Check sheet for the drawn part. Datum: minimum x, y, z corner. Units: mm. A direction names the side the tool comes from. Give positions to 0.01 mm unless a question says otherwise; leave off trailing zeros. Order: outer loops, then holes, each group sorted by start corner. A loop starts at its lowest first (then second) coordinate and runs counter-clockwise, first axis right, second up. Notation, with made-up numbers: M 26.25,0.5 L 31.25,0.5 A14 cw 31.25,4.5 Z; hole C 47,6 d10. An arc over 180 degrees is marked long. Answer in a Markdown table with one row per item. Add a question column.
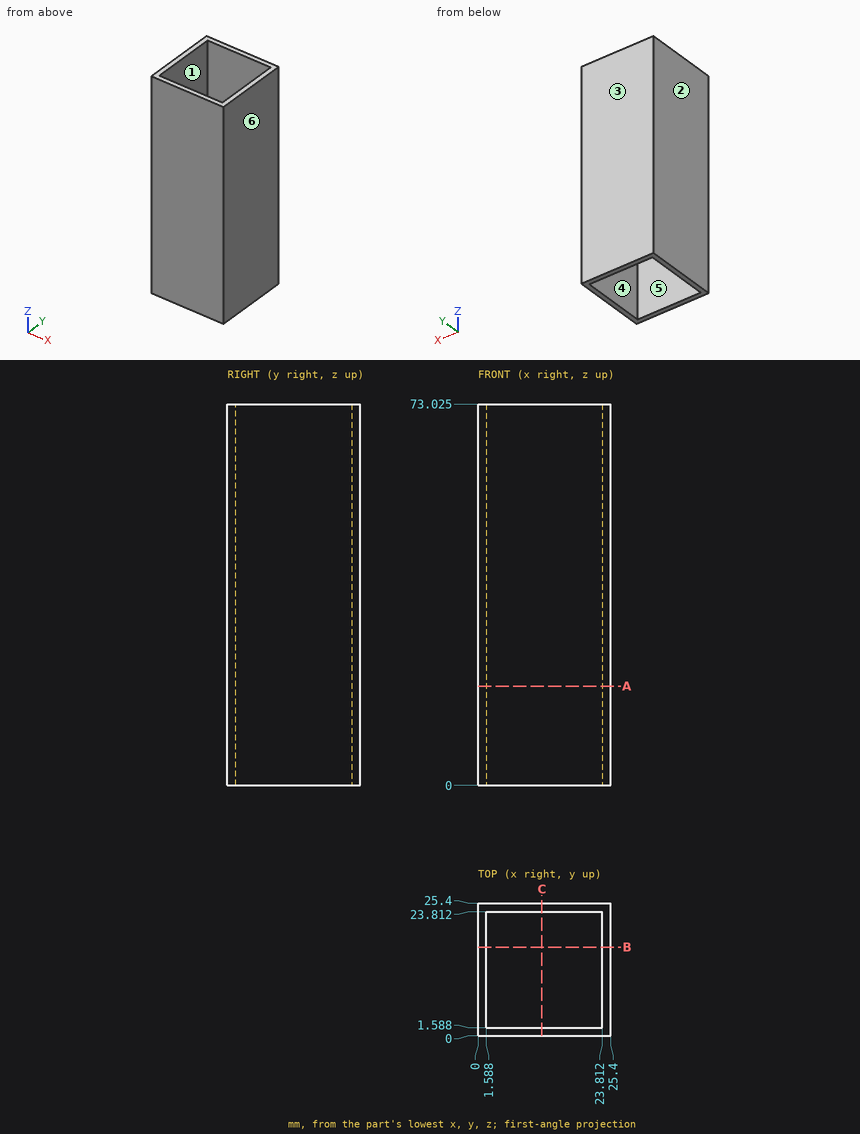
Q1. Tool access check on the marked faces 5 and 6. Record the directions out of +Z, -Z, +X, -X, +Y, -Y that give a thin tool (end or side, any length) a straight path to the whole face; none if there is none.
Q2. Thickness scan on probe 1 along X at (y, z) = (16.25, 27.5). Record the ranges inside material, lowest first.
Q3. Cross-section at A-A (z = 19). Record the boundary of the cut face in (x, y), and give its area (3 significant figures).
Q4. Draft check along Y on the marked faces 1, 2, 3 and 4. Enter one of: pulls with the +Y half, pulls with the -Y half, needs draft (parallel to the pull), parting line crosses it, or undercut.
Q5. Cross-section at B-B (y = 17). Record the boundary of the cut face in (x, z) (1 decimal), and give its area (3 significant figures).
Values follow:
| question | item | result |
|---|---|---|
| 1 | face 5 | +Z, -Z |
| 1 | face 6 | +Z, -Z, +X, +Y, -Y |
| 2 | probe 1 | 0 to 1.59, 23.81 to 25.4 |
| 3 | outline | M 0,0 L 25.4,0 L 25.4,25.4 L 0,25.4 Z; hole M 1.59,1.59 L 23.81,1.59 L 23.81,23.81 L 1.59,23.81 Z |
| 3 | area | 151 mm² |
| 4 | face 1 | undercut |
| 4 | face 2 | needs draft |
| 4 | face 3 | pulls with the +Y half |
| 4 | face 4 | undercut |
| 5 | outline | M 0,0 L 1.6,0 L 1.6,73 L 0,73 Z; M 23.8,0 L 25.4,0 L 25.4,73 L 23.8,73 Z |
| 5 | area | 232 mm² |
